Geometry check sheet. Reference: the model listing, model coordinates, mm. A direction names the side the tool comes from. Round coordinates to 2 decimals unless told otherwise and drop trailing zeros. Write each loop counter-clockwise with the first axis right and the second up, starting at its lowest first coordinate (ties: lowest second). Pieces come first, ordered by that corner, then holes.
Item 1: Scan lines: probe 1 along X at (y, z) = (0.7, 0); probe 2 along X at (y, z) = (1.85, -41.5). Record each from-to range of solid material in increasing order.
Item 2: Depth check by flat-ended pin: P1, Ø1.2, axis at x = 0.5, y = 2, coming from the +Z side; P2, Ø1.6, axis at x = -1, y = 2.5, coming from the -Z side; P3, Ø1.2, axis at y = 2.5, z = 41.5, coming from the -X side; P4, Ø2, axis at x = 32, z = -19, coming from the -Y side. Enter the tip coordinate at first touch or a pass-through.
Item 3: Access from +Z, -Z, +X, -X, +Y, -Y to the whole of each face (thin tool, end or side, straight path). Record for faces 1 (the face through (-31.985, 2.34, -28.521)), 2 (the face through (-20.12, 2.34, 34.92)), 3 (the face through (-19.27, 2.34, 38.28)), 4 (the face through (-39.16, 2.34, -22.57)).
Item 4: Cross-section at C-C (y = 2.4). State how many separate pieces and enclosed holes the cut face has, then the cut area to 3 significant figures.
Item 5: Cross-section at B-B (x = 0). Enter the section's corners in (y, z).
Item 6: Cross-section at D-D (x = 16). Enter the section's corners in (y, z), then the cut area to 3 significant figures.
Item 7: Cross-section at A-A (z = 0). Enter the section's corners in (x, y), then the cut area to 3 significant figures.
Item 8: Draft check along Z on faces 5 (the face through (-41, 3.1, 11)), 6 (the face through (22.63, 2.34, 39.127)), 7 (the face through (-28.47, 2.34, 28.52)). Enter one of: pulls with the +Z half, pulls with the -Z half, needs draft (parallel to the pull), parting line crosses it, or undercut.
from build123d import *

# Parameters (mm, degrees)
SKETCH_1_R               = 46.3
SKETCH_1_R_2             = 37.65
EXTRUDE_1_DEPTH          = 1.6
SKETCH_2_W               = 4.9
SKETCH_2_H               = 4.9
EXTRUDE_2_DEPTH          = 1.5
PATTERN_CIRCULAR_1_COUNT = 24


with BuildPart() as part:
    # 草图1 → 凸台-拉伸1 (new body)
    with BuildSketch(Plane(origin=(0, 0, 0), x_dir=(1, 0, 0), z_dir=(0, 1, 0))):
        Circle(SKETCH_1_R)
        Circle(SKETCH_1_R_2, mode=Mode.SUBTRACT)
    extrude(amount=EXTRUDE_1_DEPTH)

    # 草图2 → 凸台-拉伸2 (add)
    with BuildSketch(Plane(origin=(0, 1.6, 0), x_dir=(1, 0, 0), z_dir=(0, 1, 0))):
        with Locations((-42.75, 0)):
            Rectangle(SKETCH_2_W, SKETCH_2_H)
    extrude_2 = extrude(amount=EXTRUDE_2_DEPTH)

    # 阵列(圆周)1: 凸台-拉伸2 ×24 about axis
    pattern_circular_1_axis = Axis((0, 0, 0), (0, 1, 0))
    for i in range(1, PATTERN_CIRCULAR_1_COUNT):
        add(extrude_2.rotate(pattern_circular_1_axis, i * 360 / PATTERN_CIRCULAR_1_COUNT))


solid = part.part
Resolved:
1. probe 1: x = -46.3 to -37.65, 37.65 to 46.3
1. probe 2: x = -13.66 to -8.58, -2.45 to 2.45, 8.58 to 13.66
2. P1: stops at z = 46.3
2. P2: stops at z = -45.2
2. P3: stops at x = -13.82
2. P4: stops at y = 0
3. face 1: -X, +Y
3. face 2: +Y
3. face 3: +Z, +Y
3. face 4: -Z, -X, +Y
4. separate pieces: 24
4. enclosed holes: 0
4. area: 576 mm2
5. outline: (0, -46.3) - (1.6, -46.3) - (1.6, -45.2) - (3.1, -45.2) - (3.1, -40.3) - (1.6, -40.3) - (1.6, -37.65) - (0, -37.65) - close; (0, 37.65) - (1.6, 37.65) - (1.6, 40.3) - (3.1, 40.3) - (3.1, 45.2) - (1.6, 45.2) - (1.6, 46.3) - (0, 46.3) - close
6. outline: (0, -43.45) - (1.6, -43.45) - (1.6, -34.08) - (0, -34.08) - close; (0, 34.08) - (1.6, 34.08) - (1.6, 43.45) - (0, 43.45) - close
6. area: 30.0 mm2
7. outline: (-46.3, 0) - (-37.65, 0) - (-37.65, 1.6) - (-40.3, 1.6) - (-40.3, 3.1) - (-45.2, 3.1) - (-45.2, 1.6) - (-46.3, 1.6) - close; (37.65, 0) - (46.3, 0) - (46.3, 1.6) - (45.2, 1.6) - (45.2, 3.1) - (40.3, 3.1) - (40.3, 1.6) - (37.65, 1.6) - close
7. area: 42.4 mm2
8. face 5: needs draft
8. face 6: pulls with the +Z half
8. face 7: undercut
